Build history of the part. All positions in model axes, mm. Face numbers are marked on the shaded views. A direction names the side the tool comes from. Round coordinates to 2 decimals unless told otherwise and drop trailing zeros. Loops run counter-clockwise (first coordinate to the right, second up) from the corner with the lowest first, then second, coordinate; pieces in that order, holes last. Notation, with made-up numbers: (34, 22) - (41, 22) arc R22 cw to (41, 48) - close; hole circle Ø4 at (57, 22). An arc over 180 degrees is marked (long way). Put each result on its own line as item: value. Start each with the question number.
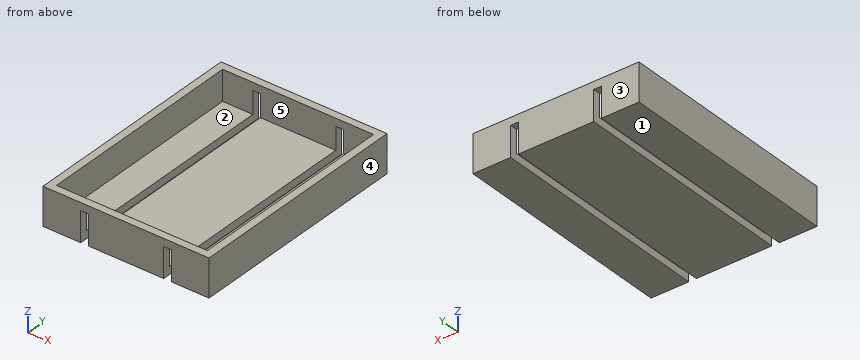
from build123d import *

# Parameters (mm, degrees)
F0_W     = 279.4
F0_H     = 381
F0_W_2   = 254
F0_H_2   = 355.6
F1_DEPTH = 50.8
F2_DEPTH = 12.7
F3_W     = 12.7
F3_H     = 381
F4_DEPTH = 50.8


with BuildPart() as f1:
    # F0 (on Top) → F1 (new body)
    with BuildSketch(Plane.XY):
        Rectangle(F0_W, F0_H)
        Rectangle(F0_W_2, F0_H_2, mode=Mode.SUBTRACT)
    extrude(amount=F1_DEPTH)

    # F0 (on Top) → F2 (join)
    with BuildSketch(Plane.XY):
        Rectangle(F0_W, F0_H)
        Rectangle(F0_W_2, F0_H_2, mode=Mode.SUBTRACT)
        Rectangle(F0_W_2, F0_H_2)
    extrude(amount=-F2_DEPTH)

    # F3 (on face) → F4 (cut)
    with BuildSketch(Plane(origin=(0, 0, -12.7), x_dir=(1, 0, 0), z_dir=(0, 0, -1))):
        with Locations((-69.85, 0)):
            Rectangle(F3_W, F3_H)
        with Locations((69.85, 0)):
            Rectangle(F3_W, F3_H)
    extrude(amount=-F4_DEPTH, mode=Mode.SUBTRACT)


solid = f1.part
1) Slice it at A-A, the plane z = -7. Write the cut outline in (x, y), and give its area (3 significant figures).
2) Drill centre lines: line 1 (X direction, y = 42, z = 17.5); line 2 (Y direction, x = -50, z = 18.5); line 3 (X direction, y = 0.5, z = -2). Where is each one in solid material? Low to high. Write a range as [from, to].
3) Slice it at B-B, the plane y = -133. Write the cut outline in (x, z), and give its area (3 significant figures).
4) Slice it at C-C, the plane z = 46. Write the cut outline in (x, y).
5) Which spindle directions (+Z, -Z, +X, -X, +Y, -Y) get a long thin tool onto all of the face, cutting with end or side? Do the marked faces 4 and 5. Say none if no direction does.
6) Pull direction Y, two halves, no side cores. Call the marked faces 1, 2 and 3: pulls with the +Y half, pulls with the -Y half, needs draft (parallel to the pull), parting line crosses it, or undercut.
7) Slice it at D-D, the plane z = 11. Write the cut outline in (x, y).
8) Drop flat-ended pins along their axis: pin 1 Ø6.5 at (x, y) = (72, -185) entering from -Z; pin 2 Ø4 at (x, y) = (-35.5, 85) entering from +Z. Give the stop position or say it passes through.
Taken from the geometry:
1. outline: (-139.7, -190.5) - (-76.2, -190.5) - (-76.2, 190.5) - (-139.7, 190.5) - close; (-63.5, -190.5) - (63.5, -190.5) - (63.5, 190.5) - (-63.5, 190.5) - close; (76.2, -190.5) - (139.7, -190.5) - (139.7, 190.5) - (76.2, 190.5) - close
1. area: 96,800 mm2
2. line 1: x = [-139.7, -127], [127, 139.7]
2. line 2: y = [-190.5, -177.8], [177.8, 190.5]
2. line 3: x = [-139.7, -76.2], [-63.5, 63.5], [76.2, 139.7]
3. outline: (-139.7, -12.7) - (-76.2, -12.7) - (-76.2, 0) - (-127, 0) - (-127, 50.8) - (-139.7, 50.8) - close; (-63.5, -12.7) - (63.5, -12.7) - (63.5, 0) - (-63.5, 0) - close; (76.2, -12.7) - (139.7, -12.7) - (139.7, 50.8) - (127, 50.8) - (127, 0) - (76.2, 0) - close
3. area: 4,520 mm2
4. outline: (-139.7, -190.5) - (139.7, -190.5) - (139.7, 190.5) - (-139.7, 190.5) - close; hole (-127, -177.8) - (127, -177.8) - (127, 177.8) - (-127, 177.8) - close
5. face 4: +Z, -Z, +X, +Y, -Y
5. face 5: +Z
6. face 1: needs draft
6. face 2: undercut
6. face 3: pulls with the +Y half
7. outline: (-139.7, -190.5) - (-76.2, -190.5) - (-76.2, -177.8) - (-127, -177.8) - (-127, 177.8) - (-76.2, 177.8) - (-76.2, 190.5) - (-139.7, 190.5) - close; (-63.5, -190.5) - (63.5, -190.5) - (63.5, -177.8) - (-63.5, -177.8) - close; (-63.5, 177.8) - (63.5, 177.8) - (63.5, 190.5) - (-63.5, 190.5) - close; (76.2, -190.5) - (139.7, -190.5) - (139.7, 190.5) - (76.2, 190.5) - (76.2, 177.8) - (127, 177.8) - (127, -177.8) - (76.2, -177.8) - close
8. pin 1: stops at z = 38.1
8. pin 2: stops at z = 0
